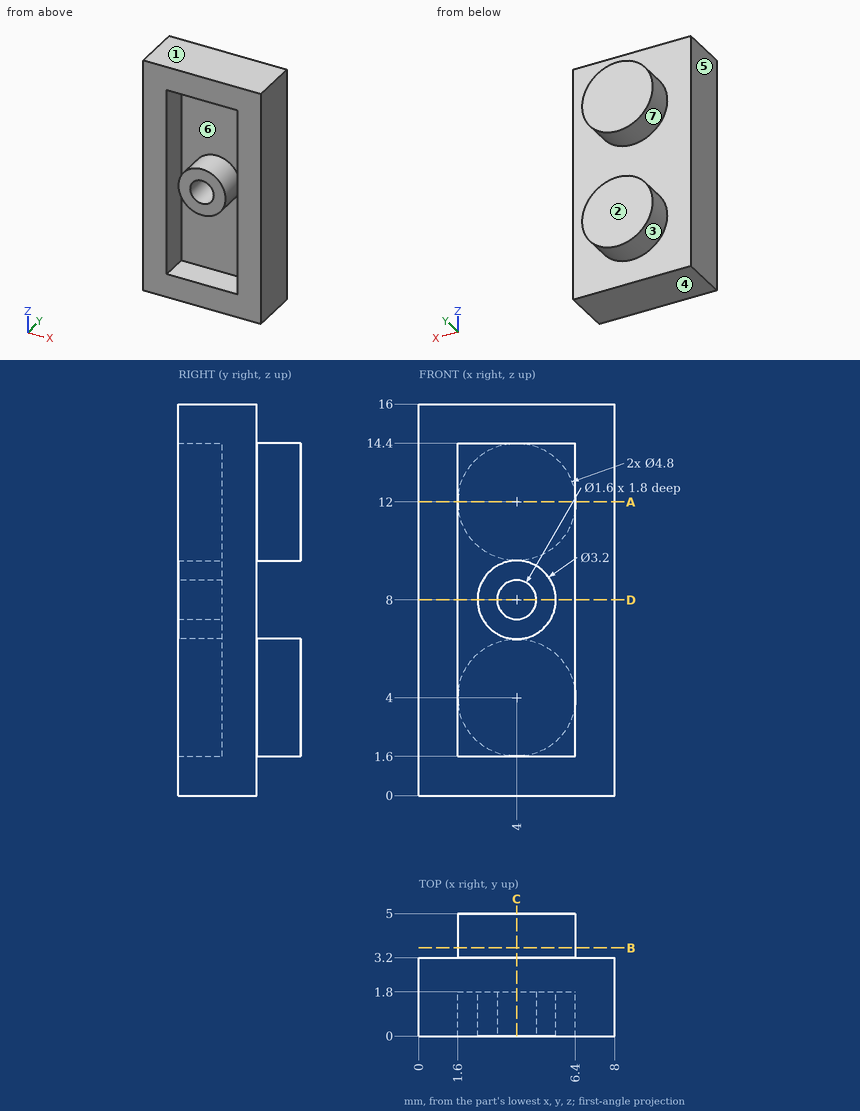
Can you work these out from the drawing? Everything is in mm from the part's minimum corner. A direction names the side the tool comes from. Coordinates: 2 decimals unless noted, no trailing zeros. Loops run counter-clockwise (first coordinate to the right, second up) from the corner with the lowest first, then second, coordinate; pieces in that order, holes last. Notation, with made-up numbers: (20, 22) -> (59, 22) arc R7 ccw to (59, 34) -> close; hole circle Ø1 at (-16.5, 64). An arc over 180 degrees is marked (long way). Return JSON: item names as keys, results as strings.
1) I need wall thicknesses on line 1 (X direction, y = 0.9, z = 8); line 2 (X direction, y = 1.75, z = 2.5); line 3 (Z direction, x = 1.75, y = 0.3). Which ranges of each line are inside material? Lowest first, please. Write a range as from..to.
Results below:
{"line 1": "0..1.6, 2.4..3.2, 4.8..5.6, 6.4..8", "line 2": "0..1.6, 6.4..8", "line 3": "0..1.6, 14.4..16"}
2) Will these pins go through, and if not, where does the flat tip stop? pin 1 (0.5 mm diameter, centred on x = 4, z = 8, fed in from -Y); pin 2 (1 mm diameter, centred on x = 5.5, z = 8, fed in from +Y).
Results below:
{"pin 1": "y = 1.8", "pin 2": "y = 3.2"}
3) If we section it at A-A, the plane z = 12: Write out the boundary of the cut face in (x, y), then the cut area to 3 significant figures.
Results below:
{"outline": "(0, 0) -> (1.6, 0) -> (1.6, 1.8) -> (6.4, 1.8) -> (6.4, 0) -> (8, 0) -> (8, 3.2) -> (6.4, 3.2) -> (6.4, 5) -> (1.6, 5) -> (1.6, 3.2) -> (0, 3.2) -> close", "area": "25.6 mm²"}
4) For the marked faces 5, 6 and 7, which set-ups out of +Z, -Z, +X, -X, +Y, -Y let a thin tool reach every point of the face, with its end or its side?
Results below:
{"face 5": "+Z, -Z, -X, +Y, -Y", "face 6": "-Y", "face 7": "+Y"}
5) If we section it at D-D, the plane z = 8: Write out the boundary of the cut face in (x, y).
Results below:
{"outline": "(0, 0) -> (1.6, 0) -> (1.6, 1.8) -> (2.4, 1.8) -> (2.4, 0) -> (3.2, 0) -> (3.2, 1.8) -> (4.8, 1.8) -> (4.8, 0) -> (5.6, 0) -> (5.6, 1.8) -> (6.4, 1.8) -> (6.4, 0) -> (8, 0) -> (8, 3.2) -> (0, 3.2) -> close"}
6) Thinking about a two-plate mould opening in Z: for the marked faces 1, 2, 3 and 4, which applies, +Z half, -Z half, draft (parallel to the pull), parting line (faces both ways), or undercut?
Results below:
{"face 1": "+Z half", "face 2": "draft", "face 3": "undercut", "face 4": "-Z half"}
7) If we section it at C-C, the plane x = 4: Write out the boundary of the cut face in (y, z), then the cut area to 3 significant figures.
Results below:
{"outline": "(0, 0) -> (3.2, 0) -> (3.2, 1.6) -> (5, 1.6) -> (5, 6.4) -> (3.2, 6.4) -> (3.2, 9.6) -> (5, 9.6) -> (5, 14.4) -> (3.2, 14.4) -> (3.2, 16) -> (0, 16) -> (0, 14.4) -> (1.8, 14.4) -> (1.8, 9.6) -> (0, 9.6) -> (0, 8.8) -> (1.8, 8.8) -> (1.8, 7.2) -> (0, 7.2) -> (0, 6.4) -> (1.8, 6.4) -> (1.8, 1.6) -> (0, 1.6) -> close", "area": "48.3 mm²"}
8) If we section it at B-B, the plane y = 3.6: Write out the boundary of the cut face in (x, z), then the cut area to 3 significant figures.
Results below:
{"outline": "circle Ø4.8 at (4, 4); circle Ø4.8 at (4, 12)", "area": "36.2 mm²"}
